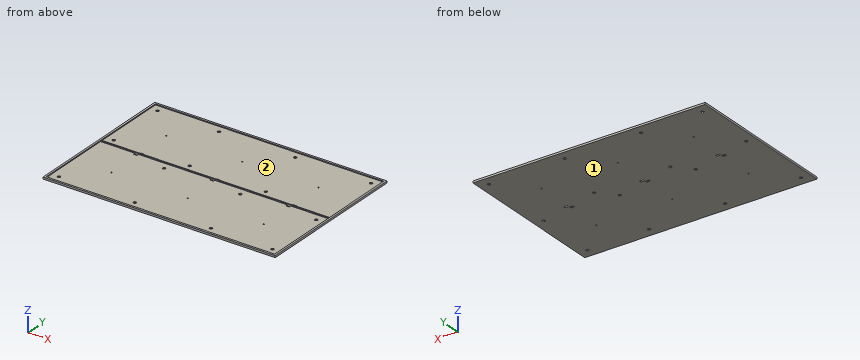
```python
from build123d import *
from build123d import SkipClean  # not in build123d's __all__

# Parameters (mm, degrees)
F0_W     = 244.15
F0_H     = 165.1
F1_DEPTH = 2
F3_DEPTH = 1
F4_R     = 1.55
F4_R_2   = 0.65
F4_W     = 3.9
F4_H     = 2.115
F5_DEPTH = 1.001


with BuildPart() as f1:
    # F0 (on Top) → F1 (new body)
    with BuildSketch(Plane.XY):
        Rectangle(F0_W, F0_H)
    extrude(amount=F1_DEPTH)

    # F2 (on face) → F3 (cut)
    with BuildSketch(Plane.XY.offset(2)):
        Polygon((120.075, 80.55), (-120.075, 80.55), (-120.075, 1), (-120.075, 0.5), (120.075, 0.5), (120.075, 1), align=None)
        Polygon((-120.075, -80.55), (120.075, -80.55), (120.075, -1), (120.075, -0.5), (-120.075, -0.5), (-120.075, -1), align=None)
    extrude(amount=-F3_DEPTH, mode=Mode.SUBTRACT)

    # F4 (on face) → F5 (cut, through all)
    with BuildSketch(Plane.XY.offset(1)):
        with Locations((-47.6721085759, 72.8278914241)):
            Circle(F4_R)
        with Locations((32.3278905301, 72.8278914241)):
            Circle(F4_R)
        with Locations((112.3278914241, 72.8278914241)):
            Circle(F4_R)
        with Locations((-112.3278914241, 8.1721085759)):
            Circle(F4_R)
        with Locations((-32.3278914241, 8.1721085759)):
            Circle(F4_R)
        with Locations((47.6721076818, 8.1721085759)):
            Circle(F4_R)
        with Locations((-80, 40.5)):
            Circle(F4_R_2)
        with Locations((-4.47e-07, 40.5)):
            Circle(F4_R_2)
        with Locations((79.999999553, 40.5)):
            Circle(F4_R_2)
        with Locations((-112.3278914241, -72.8278914241)):
            Circle(F4_R)
        with Locations((-32.3278914241, -72.8278914241)):
            Circle(F4_R)
        with Locations((47.6721076818, -72.8278914241)):
            Circle(F4_R)
        with Locations((112.3278914241, -8.1721085759)):
            Circle(F4_R)
        with Locations((32.3278905301, -8.1721085759)):
            Circle(F4_R)
        with Locations((-47.6721085759, -8.1721085759)):
            Circle(F4_R)
        with Locations((-4.47e-07, -40.5)):
            Circle(F4_R_2)
        with Locations((79.999999553, -40.5)):
            Circle(F4_R_2)
        with Locations((112.3278914241, -72.8278914241)):
            Circle(F4_R)
        with Locations((-112.3278914241, 72.8278914241)):
            Circle(F4_R)
        with Locations((-80, -40.5)):
            Circle(F4_R_2)
        with Locations((-81.949996841, -1.5575)):
            Rectangle(F4_W, F4_H)
        with Locations((-78.0499982119, 1.5575)):
            Rectangle(F4_W, F4_H)
        with Locations((-1.9499991059, -1.5575001072)):
            Rectangle(F4_W, F4_H)
        with Locations((1.9499995232, 1.5575)):
            Rectangle(F4_W, F4_H)
        with Locations((78.0497357585, -1.5575)):
            Rectangle(F4_W, F4_H)
        with Locations((81.9497343876, 1.5575)):
            Rectangle(F4_W, F4_H)
    with SkipClean():  # cleaning this boolean's faces spoils the solid; the shape is the same uncleaned
        extrude(amount=-F5_DEPTH, mode=Mode.SUBTRACT)


solid = f1.part
```
Here's how the part is built. I have some questions about the finished solid (model axes, mm). Face numbers are marked on the shaded views. Give positions to 0.01 mm unless a question says otherwise; leave off trailing zeros. Write each loop counter-clockwise with the first axis right and the second up, starting at its lowest first coordinate (ties: lowest second). Pieces come first, ordered by that corner, then holes.
(1) Imagine slicing it at A-A, the plane y = -37. Write out the boundary of the cut face in (x, z) (3 decimals), and give its area (3 significant figures).
Output values:
outline: (-122.075, 0) - (122.075, 0) - (122.075, 2) - (120.075, 2) - (120.075, 1) - (-120.075, 1) - (-120.075, 2) - (-122.075, 2) - close
area: 248 mm2
(2) Imagine slicing it at B-B, the plane x = -13.5. Write out the boundary of the cut face in (y, z), and give its area (3 significant figures).
Output values:
outline: (-82.55, 0) - (82.55, 0) - (82.55, 2) - (80.55, 2) - (80.55, 1) - (0.5, 1) - (0.5, 2) - (-0.5, 2) - (-0.5, 1) - (-80.55, 1) - (-80.55, 2) - (-82.55, 2) - close
area: 170 mm2
(3) Thinking about a two-plate mould opening in Y: for the marked faces 1 and 2, which applies, pulls with the +Y half, pulls with the -Y half, needs draft (parallel to the pull), parting line crosses it, or undercut?
Output values:
face 1: needs draft
face 2: undercut
(4) If I drill on L1, parallel to Y at x = 101, z = 1.55; L2, parallel to X at y = -29.5, z = 1.35 (3 decimals); L3, parallel to X at y = -40.5, z = 0.4 (3 decimals), over which ranges is the centre line in solid material (lowest first)?
Output values:
L1: y = -82.55 to -80.55, -0.5 to 0.5, 80.55 to 82.55
L2: x = -122.075 to -120.075, 120.075 to 122.075
L3: x = -122.075 to -80.65, -79.35 to -0.65, 0.65 to 79.35, 80.65 to 122.075
(5) Will these pins go through, and if not, where does the flat tip stop? pin 1 (8 mm diameter, centred on x = -7.5, y = 37, fed in from +Z); pin 2 (3 mm diameter, centred on x = -32.33, y = -72.83, fed in from -Z).
Output values:
pin 1: stops at z = 1
pin 2: passes through
